Read the model definition and answer for the solid it produces. Units are mm, in the model's axes. A direction names the side the tool comes from. Round coordinates to 2 decimals unless told otherwise and drop trailing zeros. Write each loop counter-clockwise with the first axis right and the second up, starting at its lowest first coordinate (ties: lowest second). Pieces come first, ordered by that corner, then holes.
from build123d import *

# Parameters (mm, degrees)
F0_R            = 44.9199
F1_DEPTH        = 241.3
F2_SIZE2        = 1.7014773719
F2_SIZE         = 6.35
F4_R            = 4.7625
F5_DEPTH        = 86
F5_COPIES_COUNT = 4


# Not quite as in the source:
# - a pattern or mirror of a feature is missing from the dataset's text; its kind, count and spacing are read off the source's solid


with BuildPart() as f1:
    # F0 (on Front) → F1 (new body)
    with BuildSketch(Plane.XZ):
        Circle(F0_R)
    extrude(amount=F1_DEPTH)

    # F2
    f2_edges = [f1.edges().sort_by_distance(p)[0] for p in [
        (-44.9199, -241.3, 0),
        (-44.9199, 0, 0),
    ]]
    f2_side = f1.faces().sort_by_distance((-44.9199, -120.65, 0))[0]
    chamfer(f2_edges, length=F2_SIZE, length2=F2_SIZE2, reference=f2_side)

    # F4 (on offset) → F5 (cut)
    with BuildSketch(Plane.XZ.offset(169.3)):
        with Locations((0, -48.0949)):
            Circle(F4_R)
    f5 = extrude(amount=-F5_DEPTH, mode=Mode.SUBTRACT)

    # F5_copies: F5 ×4 about axis
    f5_copies_axis = Axis((0, 0, 0), (0, 1, 0))
    for i in range(1, F5_COPIES_COUNT):
        add(f5.rotate(f5_copies_axis, i * 360 / F5_COPIES_COUNT), mode=Mode.SUBTRACT)


solid = f1.part
Q1. Flat-ended cylindrical pins translate along their axes: pin 1 Ø1.5 at (y, z) = (-46, 14.5) entering from -X; pin 2 Ø2 at (y, z) = (-141, 31.5) entering from -X; pin 3 Ø12 at (y, z) = (-178, -5) entering from -X; pin 4 Ø8 at (y, z) = (-30, 27) entering from -X. Find the tip coordinate at first contact, or state that the pin passes through.
Verdict:
pin 1: stops at x = -42.76
pin 2: stops at x = -32.98
pin 3: stops at x = -44.92
pin 4: stops at x = -38.58
Q2. Section A-A (y = -110) is taken. Determine the outline of the cut face in (x, z) (1 decimal), then the cut area to 3 significant figures.
Verdict:
outline: (-44.8, -3.4) arc R44.9 ccw to (-3.4, -44.8) arc R4.8 cw to (3.4, -44.8) arc R44.9 ccw to (44.8, -3.4) arc R4.8 cw to (44.8, 3.4) arc R44.9 ccw to (3.4, 44.8) arc R4.8 cw to (-3.4, 44.8) arc R44.9 ccw to (-44.8, 3.4) arc R4.8 cw to start
area: 6,310 mm2
Q3. Determine the mould class of faces 1 (the cylindrical face through (-0.054, -126.902, 43.333)), 2 (the flat face through (-1, 0, 1)), 3 (the cylindrical face through (-43.333, -126.902, -0.054)) for opening direction X: pulls with the +X half, pulls with the -X half, needs draft (parallel to the pull), parting line crosses it, or undercut.
Verdict:
face 1: undercut
face 2: needs draft
face 3: pulls with the -X half
Q4. Which of the six approach directions +Z, -Z, +X, -X, +Y, -Y give full straight-line access (tool end or side, diameter ignored) to faces 4 (the cylindrical face through (43.333, -126.902, 0.054)), 5 (the cylindrical face through (0.054, -126.902, -43.333)), 6 (the cylindrical face through (42.846, -119.05, 13.493))?
Verdict:
face 4: +X
face 5: -Z
face 6: +Y, -Y
Q5. Section B-B (y = -218) is taken. Determine the outline of the cut face in (x, z).
Verdict:
outline: circle Ø89.84 at (0, 0)
Q6. Straight lines are drawn through the part: probe 1 along Z at (x, y) = (-4, -185); probe 2 along Z at (x, y) = (-22, -118); probe 3 along X at (y, z) = (-66, -21). For each, find the intervals that lie inside material, in ascending order.
Verdict:
probe 1: z = -44.74 to 44.74
probe 2: z = -39.16 to 39.16
probe 3: x = -39.71 to 39.71
